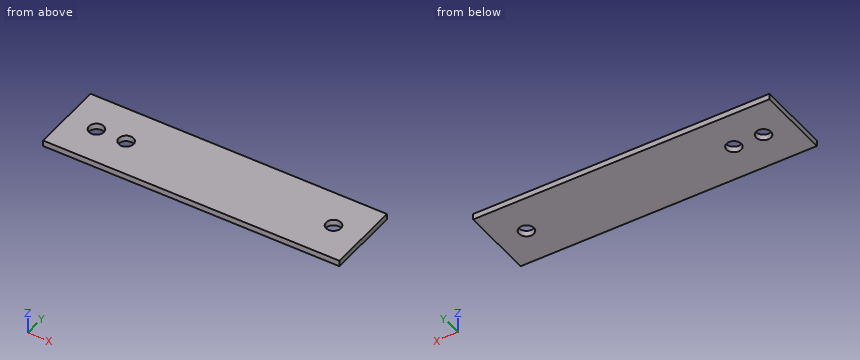
```python
from build123d import *

# Parameters (mm, degrees)
ESBO_O1_W                = 100
ESBO_O1_H                = 25
ESBO_O1_R                = 2.5
RESSALTO_EXTRUS_O1_DEPTH = 2


with BuildPart() as part:
    # Esboço1 → Ressalto-extrusão1 (new body)
    with BuildSketch(Plane.XY):
        with Locations((21.110395733, -2.804487179)):
            Rectangle(ESBO_O1_W, ESBO_O1_H)
        with Locations((-18.889604267, -2.804487179)):
            Circle(ESBO_O1_R, mode=Mode.SUBTRACT)
        with Locations((-8.889604267, -2.804487179)):
            Circle(ESBO_O1_R, mode=Mode.SUBTRACT)
        with Locations((61.110395733, -2.804487179)):
            Circle(ESBO_O1_R, mode=Mode.SUBTRACT)
    extrude(amount=RESSALTO_EXTRUS_O1_DEPTH)


solid = part.part
```
Source: CAD feature listing. Evaluate the final solid. Frame: model axes, mm. Coordinates: 2 decimals unless noted, no trailing zeros. Order: outer loops, then holes, each group sorted by start corner. A loop starts at its lowest first (then second) coordinate and runs counter-clockwise, first axis right, second up. Notation, with made-up numbers: (59, -3.5) - (96, -3.5) arc R15 ccw to (96, 25.5) - close; hole circle Ø3 at (39, 13). An arc over 180 degrees is marked (long way). One line per item, written item: value.
1) Ray query, line 1 (X direction, y = -0.5, z = 1.1); line 2 (X direction, y = -2, z = 0.7); line 3 (Y direction, x = -8.5, z = 1.55). Return the intervals inside material, ascending. Write a range as [from, to].
Computed values:
line 1: x = [-28.89, -19.86], [-17.92, -9.86], [-7.92, 60.14], [62.08, 71.11]
line 2: x = [-28.89, -21.26], [-16.52, -11.26], [-6.52, 58.74], [63.48, 71.11]
line 3: y = [-15.3, -5.27], [-0.34, 9.7]
2) Cut plane A-A on x = -18.5. Output: boundary loops of the cut face in (y, z), plus the area to 3 significant figures.
Computed values:
outline: (-15.3, 0) - (-5.27, 0) - (-5.27, 2) - (-15.3, 2) - close; (-0.34, 0) - (9.7, 0) - (9.7, 2) - (-0.34, 2) - close
area: 40.1 mm^2
3) Cut plane B-B on z = 1.45. Output: boundary loops of the cut face in (x, y).
Computed values:
outline: (-28.89, -15.3) - (71.11, -15.3) - (71.11, 9.7) - (-28.89, 9.7) - close; hole circle Ø5 at (-18.89, -2.8); hole circle Ø5 at (-8.89, -2.8); hole circle Ø5 at (61.11, -2.8)
4) Contact query for a flat-ended pin moving along its axis: pin 1 (3 mm diameter, centred on x = -8.89, y = -2.8, fed in from +Z). Output: stop coordinate, or through.
Computed values:
pin 1: passes through
